from build123d import *

# Parameters (mm, degrees)
F1_DEPTH = 51
F2_DEPTH = 2
F3_DEPTH = 23
F5_DEPTH = 10


with BuildPart() as f1:
    # F0 (on Right) → F1 (new body)
    with BuildSketch(Plane.YZ):
        Polygon((-106.4311944246, 30.6635548347), (-88.4311944246, 48.6635548347), (-70.4311944246, 30.6635548347), (-63.1831944246, 23.4155548347), (-40.4311944246, -9.4364451653), (-37.9983836671, -9.4364451653), (-61.6478004918, 24.697180939), (-88.4311944246, 51.4919819594), (-115.2145883574, 24.697180939), (-138.8640051821, -9.4364451653), (-136.4311944246, -9.4364451653), (-113.6791944246, 23.4155548347), align=None)
    extrude(amount=F1_DEPTH)

    # F2 (cut): a face of the model
    f2_faces = [f1.faces().sort_by_distance(p)[0] for p in [
        (51, -100.9894629386, 37.2615078041),
    ]]
    extrude(f2_faces, amount=-F2_DEPTH, mode=Mode.SUBTRACT)

    # F3 (add): a face of the model
    f3_faces = [f1.faces().sort_by_distance(p)[0] for p in [
        (0, -100.9894629386, 37.2615078041),
    ]]
    extrude(f3_faces, amount=F3_DEPTH)

    # F4 (on face) → F5 (join)
    with BuildSketch(Plane(origin=(-23, 0, 0), x_dir=(0, -1, 0), z_dir=(-1, 0, 0))):
        Polygon((88.4311944246, 51.4919819594), (67.6116343818, 30.6635548347), (70.4311944246, 30.6635548347), (88.4311944246, 48.6635548347), (106.4311944246, 30.6635548347), (109.2507544675, 30.6635548347), align=None)
    extrude(amount=F5_DEPTH)


solid = f1.part
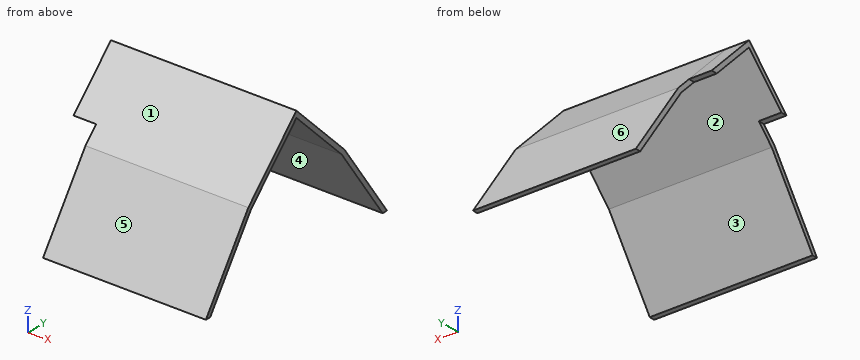
Here's how the part is built. I have some questions about the finished solid (model axes, mm). Face numbers are marked on the shaded views. A direction names the side the tool comes from. Coordinates: 2 decimals unless noted, no trailing zeros. Loops run counter-clockwise (first coordinate to the right, second up) from the corner with the lowest first, then second, coordinate; pieces in that order, holes last.
1. I need wall thicknesses on L1, parallel to Y at x = -21.5, z = 5; L2, parallel to Y at x = -5, z = 29.5; L3, parallel to Z at x = 12, y = -43. Which ranges of each line are inside material? Lowest first, please.
2. If we mould it in two halves opening along Y, with no side actions, what happens to the marked faces 3, 4, 5 and 6? For each: pulls with the +Y half, pulls with the -Y half, needs draft (parallel to the pull), parting line crosses it, or undercut.
3. Imagine slicing it at C-C, the plane z = 16. Please give me the cut outline in (x, y).
4. Imagine slicing it at A-A, the plane z = 3. Please give me the cut outline in (x, y).
5. For the marked faces 1 and 2, which set-ups out of +Z, -Z, +X, -X, +Y, -Y let a thin tool reach every point of the face, with its end or its side?
6. Imagine slicing it at D-D, the plane y = -122.5. Please give me the cut outline in (x, z).
7. For P1, Ø2.5, axis at x = -29.5, y = -69, coming from the -Z side; P2, Ø3, axis at x = 7.5, y = -80, coming from the +Z side; P3, Ø10, axis at x = 7, y = -104.5, coming from the +Z side, each with a flat end and sliding along its axis, tell me the tip position at first contact or that it passes through.
8. Imagine slicing it at B-B, the plane x = 31. Please give me the cut outline in (y, z), and give its area (3 significant figures).
Taken from the geometry:
1. L1: y = -128.86 to -126.43, -50.43 to -48
1. L2: y = -110.41 to -107.59, -69.27 to -66.45
1. L3: z = -5.73 to -2.22
2. face 3: undercut
2. face 4: undercut
2. face 5: pulls with the -Y half
2. face 6: pulls with the +Y half
3. outline: (-23, -121.24) - (49, -121.24) - (49, -118.81) - (-23, -118.81) - close; (-23, -58.05) - (49, -58.05) - (49, -55.62) - (-23, -55.62) - close
4. outline: (-23, -130.25) - (49, -130.25) - (49, -127.82) - (-23, -127.82) - close; (-23, -49.04) - (49, -49.04) - (49, -46.61) - (-23, -46.61) - close
5. face 1: +Z, +X, -X, -Y
5. face 2: -Z, +X, -X
6. outline: (-23, 10.68) - (49, 10.68) - (49, 14.18) - (-23, 14.18) - close
7. P1: stops at z = 30.66
7. P2: stops at z = 44.56
7. P3: stops at z = 40.42
8. outline: (-138.86, -9.44) - (-136.43, -9.44) - (-113.68, 23.42) - (-88.43, 48.66) - (-63.18, 23.42) - (-40.43, -9.44) - (-38, -9.44) - (-61.65, 24.7) - (-88.43, 51.49) - (-115.21, 24.7) - close
8. area: 310 mm2
